Here's how the part is built. I have some questions about the finished solid (model axes, mm). Face numbers are marked on the shaded views. A direction names the side the tool comes from. Coordinates: 2 decimals unless noted, no trailing zeros. Write each loop counter-clockwise with the first axis right and the second up, starting at its lowest first coordinate (ties: lowest second). Pieces come first, ordered by that corner, then holes.
```python
from build123d import *

# Parameters (mm, degrees)
F0_W      = 720
F0_H      = 300
F1_DEPTH  = 25
F2_W      = 50
F2_H      = 50
F3_DEPTH  = 100
F4_W      = 50
F4_H      = 50
F5_DEPTH  = 100
F6_W      = 50
F6_H      = 50
F7_DEPTH  = 25
F8_R      = 25
F9_DEPTH  = 150
F10_W     = 45
F10_H     = 106.833779
F11_DEPTH = 150
F13_DEPTH = 50
F14_W     = 70
F14_H     = 70
F15_DEPTH = 150
F16_DEPTH = 130
F17_R     = 25
F18_W     = 150
F18_H     = 120
F19_DEPTH = 25
F20_W     = 104
F20_H     = 100
F21_DEPTH = 150
F22_W     = 104
F22_H     = 170
F23_DEPTH = 25
F24_W     = 20
F24_H     = 71.34236
F25_DEPTH = 80
F26_R     = 7.5
F27_DEPTH = 616.001
F28_W     = 58.787813
F28_H     = 143
F29_DEPTH = 10


with BuildPart() as f1:
    # F0 (on Top) → F1 (new body)
    with BuildSketch(Plane.XY):
        Rectangle(F0_W, F0_H)
    extrude(amount=F1_DEPTH)

    # F2 (on face) → F3 (join)
    with BuildSketch(Plane.XY.offset(25)):
        with Locations((-335, -125)):
            Rectangle(F2_W, F2_H)
    extrude(amount=F3_DEPTH)

    # F4 (on face) → F5 (join)
    with BuildSketch(Plane.XY.offset(25)):
        with Locations((335, -125)):
            Rectangle(F4_W, F4_H)
        with Locations((-335, 125)):
            Rectangle(F4_W, F4_H)
        with Locations((335, 125)):
            Rectangle(F4_W, F4_H)
    extrude(amount=F5_DEPTH)

    # F6 (on face) → F7 (join)
    with BuildSketch(Plane.XY.offset(125)):
        with Locations((-335, 125)):
            Rectangle(F6_W, F6_H)
        Polygon((360, 150), (-310, 150), (-310, 100), (-360, 100), (-360, -150), (360, -150), align=None)
    extrude(amount=F7_DEPTH)

    # F8 (on face) → F9 (join)
    with BuildSketch(Plane.XY.offset(150)):
        with Locations((-310, 0)):
            Circle(F8_R)
    extrude(amount=F9_DEPTH)

    # F10 (on face) → F11 (join)
    with BuildSketch(Plane.XY.offset(150)):
        with Locations((106.5, -53.416889)):
            Rectangle(F10_W, F10_H)
        with Locations((106.5, 53.416889)):
            Rectangle(F10_W, F10_H)
    extrude(amount=F11_DEPTH)

    # F12 (on face) → F13 (cut)
    with BuildSketch(Plane.YZ.offset(129)):
        Polygon((81.833779, 300), (-81.833779, 300), (-81.833779, 221.944749), (-21.833779, 234.489977), (0, 209.399506), (21.833779, 234.489977), (81.833779, 221.944749), align=None)
    extrude(amount=-F13_DEPTH, mode=Mode.SUBTRACT)

    # F14 (on face) → F15 (join)
    with BuildSketch(Plane.XY.offset(150)):
        with Locations((221, 185)):
            Rectangle(F14_W, F14_H)
    extrude(amount=-F15_DEPTH)

    # F14 (on face) → F16 (join)
    with BuildSketch(Plane.XY.offset(150)):
        with Locations((221, 185)):
            Rectangle(F14_W, F14_H)
    extrude(amount=F16_DEPTH)

    # F17
    f17_edges = [f1.edges().sort_by_distance(p)[0] for p in [
        (-335, 0, 300),
    ]]
    fillet(f17_edges, radius=F17_R)

    # F18 (on face) → F19 (cut)
    with BuildSketch(Plane.XY.offset(150)):
        with Locations((285, -10)):
            Rectangle(F18_W, F18_H)
    extrude(amount=-F19_DEPTH, mode=Mode.SUBTRACT)

    # F20 (on face) → F21 (cut)
    with BuildSketch(Plane.XY.offset(150)):
        with Locations((308, 100)):
            Rectangle(F20_W, F20_H)
    extrude(amount=-F21_DEPTH, mode=Mode.SUBTRACT)

    # F22 (on face) → F23 (join)
    with BuildSketch(Plane.XY.offset(25)):
        with Locations((308, 135)):
            Rectangle(F22_W, F22_H)
    extrude(amount=-F23_DEPTH)

    # F24 (on face) → F25 (cut)
    with BuildSketch(Plane.XZ.offset(-150)):
        with Locations((221, 244.32882)):
            Rectangle(F24_W, F24_H)
    extrude(amount=-F25_DEPTH, mode=Mode.SUBTRACT)

    # F26 (on face) → F27 (cut, through all)
    with BuildSketch(Plane.YZ.offset(256)):
        with Locations((185, 255.659133)):
            Circle(F26_R)
    extrude(amount=-F27_DEPTH, mode=Mode.SUBTRACT)

    # F28 (on face) → F29 (join)
    with BuildSketch(Plane.XY.offset(25)):
        with Locations((330.606093, 98.5)):
            Rectangle(F28_W, F28_H)
    extrude(amount=F29_DEPTH)


solid = f1.part
```
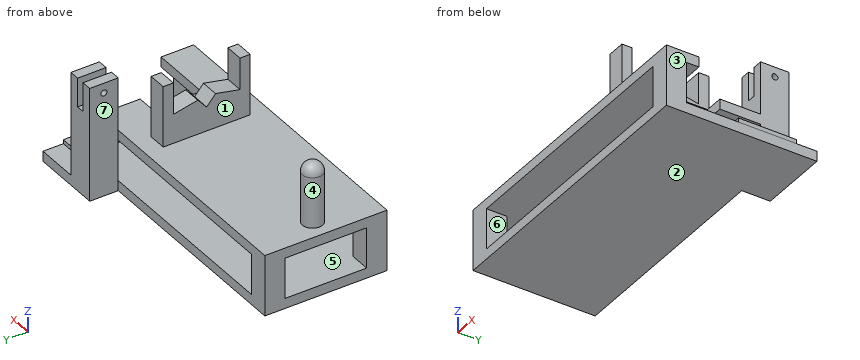
1) Imagine slicing it at B-B on y = 185. Please give me the cut outline in (x, z).
Values follow:
outline: (186, 0) - (360, 0) - (360, 25) - (256, 25) - (256, 248.16) - (231, 248.16) - (231, 208.66) - (211, 208.66) - (211, 248.16) - (186, 248.16) - close; (186, 263.16) - (211, 263.16) - (211, 280) - (186, 280) - close; (231, 263.16) - (256, 263.16) - (256, 280) - (231, 280) - close
2) On a 3-axis mill with a long thin cutter (end or side, diameter ignored), from which of +Z, -Z, +X, -X, +Y, -Y can I reach the whole of each face in a straight line? I mean the marked faces 4, 5, 6 and 7. Say none if no direction works.
Values follow:
face 4: +Z
face 5: none
face 6: +Y, -Y
face 7: +Z, -Z, -X, +Y
3) We'd pull the mould along X, two halves only. Please class the marked faces 1, 2 and 3: pulls with the +X half, pulls with the -X half, needs draft (parallel to the pull), parting line crosses it, or undercut.
Values follow:
face 1: undercut
face 2: needs draft
face 3: pulls with the +X half
4) Imagine slicing it at C-C on z = 162.5. Please give me the cut outline in (x, y), then the cut area to 3 significant figures.
Values follow:
outline: circle Ø50 at (-310, 0); (84, -106.83) - (129, -106.83) - (129, 106.83) - (84, 106.83) - close; (186, 150) - (256, 150) - (256, 220) - (186, 220) - close
area: 16,500 mm2
5) Will these pins go through, and if not, where does the flat tip stop? pin 1 (13.5 mm diameter, centred on x = 105, z = 280.5, fed in from -Y); pin 2 (1 mm diameter, centred on x = 25.5, y = -107.5, fed in from +Z); pin 3 (20 mm diameter, centred on x = 307, z = 140.5, fed in from +Y).
Values follow:
pin 1: stops at y = -106.83
pin 2: stops at z = 150
pin 3: stops at y = -70
6) I need wall thicknesses on probe 1 along Z at (x, y) = (-50, -123.5); probe 2 along Z at (x, y) = (238.5, 185); probe 3 along Y at (x, z) = (247, 218). Which ranges of each line are inside material? Lowest first, please.
Values follow:
probe 1: z = 0 to 25, 125 to 150
probe 2: z = 0 to 248.16, 263.16 to 280
probe 3: y = 150 to 220
7) Imagine slicing it at D-D on y = -126. Please give me the cut outline in (x, z), then the cut area to 3 significant figures.
Values follow:
outline: (-360, 0) - (360, 0) - (360, 150) - (-360, 150) - close; hole (-310, 25) - (310, 25) - (310, 125) - (-310, 125) - close
area: 46,000 mm2
8) Imagine slicing it at A-A on x = -194. Please give me the cut outline in (y, z).
Values follow:
outline: (-150, 0) - (150, 0) - (150, 25) - (-150, 25) - close; (-150, 125) - (150, 125) - (150, 150) - (-150, 150) - close
